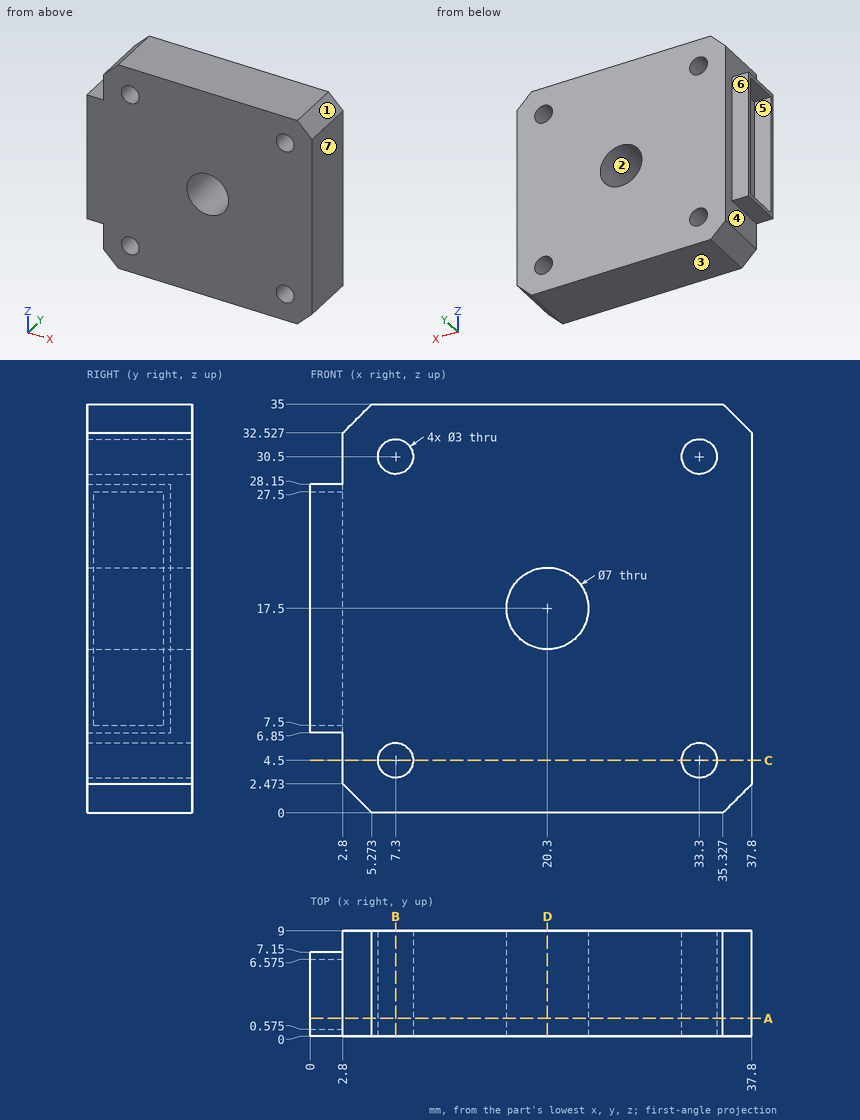
Geometry: see drawing. Coordinates: mm, zero at the bounding-box minimum. A direction names the side the tool comes from. Round coordinates to 2 decimals unless told otherwise and drop trailing zeros. Write each loop counter-clockwise with the first axis right and the second up, starting at its lowest first coordinate (ties: lowest second). Pieces come first, ordered by that corner, then holes.
Item 1: Section query C-C (z = 4.5). Return loops of the section in (x, y).
Item 2: Section query A-A (y = 1.5). Return loops of the section in (x, z), plus the area to 3 significant figures.
Item 3: Set-up query: the marked faces 5, 6 and 7. Return all of +Z, -Z, +X, -X, +Y, -Y with unobstructed straight access to the full face (end or side cutting, diameter ignored); none if empty.
Item 4: Pin query (flat end, axial travel): P1, Ø4, axis at x = 7.3, z = 30.5, coming from the -Y side; P2, Ø0.8, axis at x = 2, z = 13.5, coming from the +Y side; P3, Ø0.8, axis at x = 1, y = 2.5, coming from the -Z side; P4, Ø1.4, axis at x = 1, y = 3, coming from the +Z side. Return the tip coordinate at first contact, or that it passes through.
Item 5: Section query B-B (x = 7.3). Return loops of the section in (y, z), plus the area to 3 significant figures.
Item 6: Mould query, pull axis Z, two halves, no side actions, for the marked faces 1, 2, 3 and 4. Classes: +Z half, -Z half, draft (parallel to the pull), parting line (faces both ways), or undercut.
Item 7: Section query D-D (x = 20.3). Return loops of the section in (y, z), plus the area to 3 significant figures.
Item 8: Material intervals for L1, parallel to Z at x = 7.3, y = 6.25; L2, parallel to X at y = 2, z = 4.5; L3, parallel to X at y = 4.5, z = 30, sorted ascending.
Completed:
1. outline: (2.8, 0) - (5.8, 0) - (5.8, 9) - (2.8, 9) - close; (8.8, 0) - (31.8, 0) - (31.8, 9) - (8.8, 9) - close; (34.8, 0) - (37.8, 0) - (37.8, 9) - (34.8, 9) - close
2. outline: (0, 6.85) - (2.8, 6.85) - (2.8, 2.47) - (5.27, 0) - (35.33, 0) - (37.8, 2.47) - (37.8, 32.53) - (35.33, 35) - (5.27, 35) - (2.8, 32.53) - (2.8, 28.15) - (0, 28.15) - (0, 27.5) - (2.8, 27.5) - (2.8, 7.5) - (0, 7.5) - close; hole circle Ø3 at (7.3, 4.5); hole circle Ø3 at (7.3, 30.5); hole circle Ø7 at (20.3, 17.5); hole circle Ø3 at (33.3, 4.5); hole circle Ø3 at (33.3, 30.5)
2. area: 1,150 mm2
3. face 5: -X
3. face 6: +Z, -Z, -X, +Y
3. face 7: +Z, -Z, +X, +Y, -Y
4. P1: stops at y = 0
4. P2: stops at y = 7.15
4. P3: stops at z = 6.85
4. P4: stops at z = 28.15
5. outline: (0, 0) - (9, 0) - (9, 3) - (0, 3) - close; (0, 6) - (9, 6) - (9, 29) - (0, 29) - close; (0, 32) - (9, 32) - (9, 35) - (0, 35) - close
5. area: 261 mm2
6. face 1: +Z half
6. face 2: undercut
6. face 3: -Z half
6. face 4: draft
7. outline: (0, 0) - (9, 0) - (9, 14) - (0, 14) - close; (0, 21) - (9, 21) - (9, 35) - (0, 35) - close
7. area: 252 mm2
8. L1: z = 0 to 3, 6 to 29, 32 to 35
8. L2: x = 2.8 to 5.8, 8.8 to 31.8, 34.8 to 37.8
8. L3: x = 2.8 to 5.89, 8.71 to 31.89, 34.71 to 37.8
